Part print with two shaded views. Sizes in mm from the minimum x, y, z corner. A direction names the side the tool comes from. Coordinates: 2 decimals unless noted, no trailing zeros. Order: outer loops, then holes, each group sorted by start corner. A loop starts at its lowest first (then second) coordinate and runs counter-clockwise, first axis right, second up.
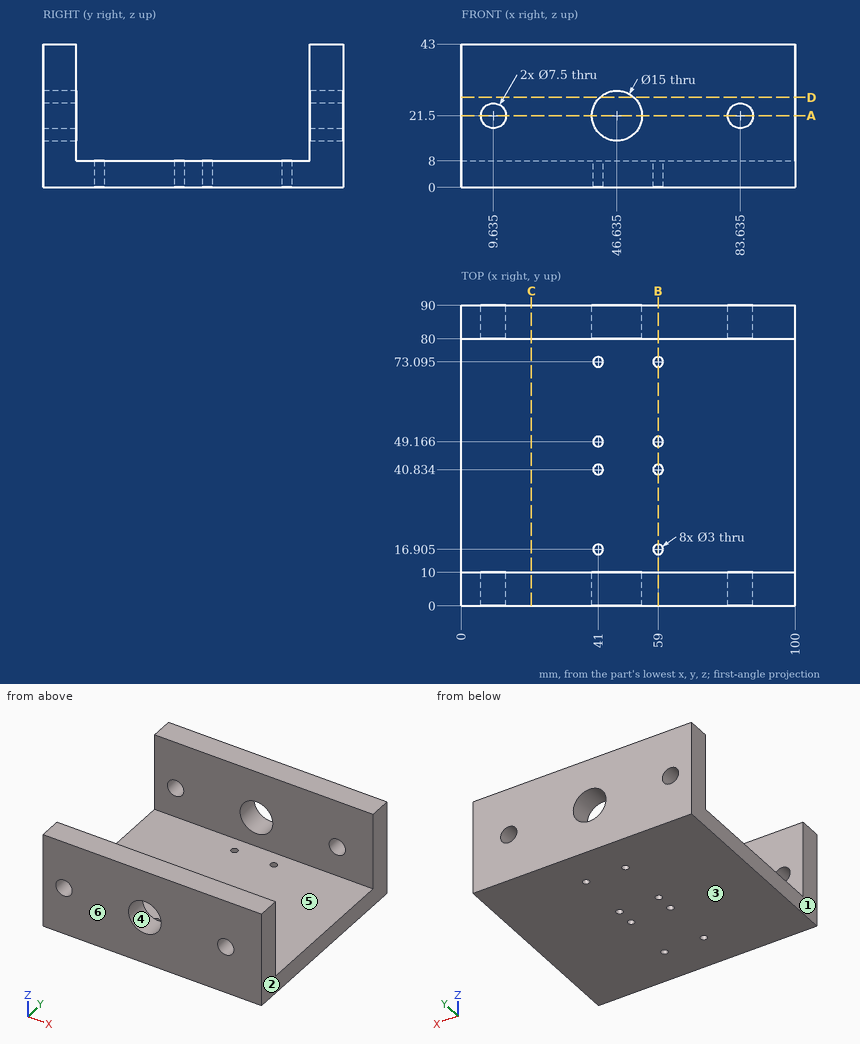
Q1. Mould opens along X. For the marked faces 1, 2, 3 and 4 say: pulls with the +X half, pulls with the -X half, needs draft (parallel to the pull), parting line crosses it, or undercut.
Results list:
face 1: pulls with the -X half
face 2: pulls with the +X half
face 3: needs draft
face 4: undercut
Q2. Cut at D-D on z = 27. Write the cut outline in (x, y), and give its area (3 significant figures).
Results list:
outline: (0, 0) - (41.54, 0) - (41.54, 10) - (0, 10) - close; (0, 80) - (41.54, 80) - (41.54, 90) - (0, 90) - close; (51.73, 0) - (100, 0) - (100, 10) - (51.73, 10) - close; (51.73, 80) - (100, 80) - (100, 90) - (51.73, 90) - close
area: 1,800 mm2
Q3. Wall check: line 1 along X through (y, z) = (5.75, 21.5) (1 decimal); line 2 along Y through (x, z) = (59, 6.25) (1 decimal); line 3 along Y through (x, z) = (41.5, 31). Give the ranges that are in metal, low to high.
Results list:
line 1: x = 0 to 5.9, 13.4 to 39.1, 54.1 to 79.9, 87.4 to 100
line 2: y = 0 to 15.4, 18.4 to 39.3, 42.3 to 47.7, 50.7 to 71.6, 74.6 to 90
line 3: y = 0 to 10, 80 to 90
Q4. Which spindle directions (+Z, -Z, +X, -X, +Y, -Y) get a long thin tool onto all of the face, cutting with end or side? Do the marked faces 5 and 6. Say none if no direction does.
Results list:
face 5: +Z, +X, -X
face 6: +Z, -Z, +X, -X, -Y
Q5. Cut at B-B on x = 59. Write the cut outline in (y, z) (1 decimal).
Results list:
outline: (0, 0) - (15.4, 0) - (15.4, 8) - (10, 8) - (10, 43) - (0, 43) - close; (18.4, 0) - (39.3, 0) - (39.3, 8) - (18.4, 8) - close; (42.3, 0) - (47.7, 0) - (47.7, 8) - (42.3, 8) - close; (50.7, 0) - (71.6, 0) - (71.6, 8) - (50.7, 8) - close; (74.6, 0) - (90, 0) - (90, 43) - (80, 43) - (80, 8) - (74.6, 8) - close
Q6. Cut at C-C on x = 21. Write the cut outline in (y, z), and give its area (3 significant figures).
Results list:
outline: (0, 0) - (90, 0) - (90, 43) - (80, 43) - (80, 8) - (10, 8) - (10, 43) - (0, 43) - close
area: 1,420 mm2
Q7. Pin check, flat tips, straight feed: pin 1 Ø4 at (x, y) = (41, 73.09) entering from +Z; pin 2 Ø10 at (x, z) = (74, 22) entering from -Y. Stop position of each tip, or through.
Results list:
pin 1: stops at z = 8
pin 2: stops at y = 0
Q8. Cut at A-A on z = 21.5. Count the separate pieces of the cut face and the enclosed holes in it, and give its area (3 significant figures).
Results list:
separate pieces: 8
enclosed holes: 0
area: 1,400 mm2
